The listing builds one solid part. Answer for the finished solid, in the listing's coordinates (mm). Face numbers are marked on the shaded views. A direction names the side the tool comes from. Give positions to 0.01 mm unless a question says otherwise; leave off trailing zeros. Loops run counter-clockwise (first coordinate to the right, second up) from the corner with the lowest first, then second, coordinate; pieces in that order, holes last. Notation, with made-up numbers: (58.5, 36.5) - (94.5, 36.5) arc R21 cw to (94.5, 75.5) - close; hole circle Ø8 at (62.25, -16.5). An arc over 180 degrees is marked (long way). Answer as CSV lines item,"result". Start each with the question number.
1) A cutting plane is placed at A-A (z = 13.5). Determine the outline of the cut face in (x, y).
2) Find the intervals of material crossed by line 1 along X through (y, z) = (-2, 17.5); line 2 along Z through (x, y) = (11, 22); line 3 along X through (y, z) = (-4, 10), in increasing order.
3) A cutting plane is placed at B-B (x = -12). Determine the outline of the cut face in (y, z), and give its area (3 significant figures).
4) For a pull along Y with two mould halves and no side action, classify the marked faces 1, 2 and 3 as pulls with the +Y half, pulls with the -Y half, needs draft (parallel to the pull), parting line crosses it, or undercut.
5) Flat-ended cylindrical pins translate along their axes: pin 1 (12.5 mm diameter, centred on x = 0, y = 0.19, fed in from +Z); pin 2 (1.5 mm diameter, centred on x = 12.5, y = -15, fed in from +Z); pin 3 (10 mm diameter, centred on y = -6, z = 6.5, fed in from -X); pin 4 (6 mm diameter, centred on x = 35, y = 0, fed in from +Z). Find the tip coordinate at first contact, or state that the pin passes through.
6) For the marked faces 4 and 5, determine the directions among +Z, -Z, +X, -X, +Y, -Y from which every point of the face is accessible in a straight line to the end or side of a thin tool.
7) A cutting plane is placed at D-D (x = -35). Determine the outline of the cut face in (y, z), and give its area (3 significant figures).
8) A cutting plane is placed at C-C (y = -11). Determine the outline of the cut face in (x, z), and give its area (3 significant figures).
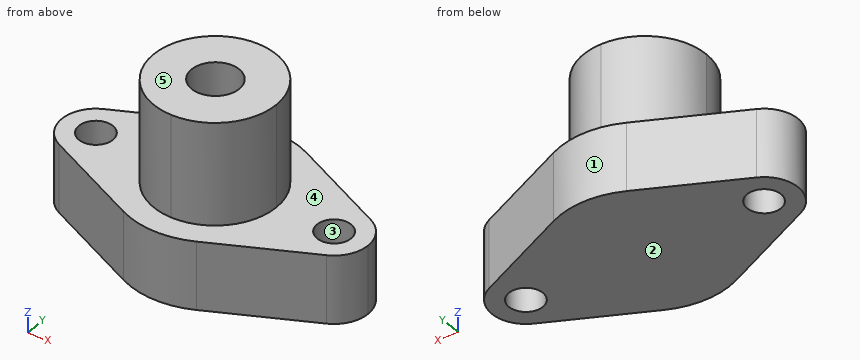
```python
from build123d import *

# Parameters (mm, degrees)
F1_DEPTH = 20
F3_D     = 10
F4_DEPTH = 30
F6_D     = 14
F6_DEPTH = 25
F6_TIP   = 4.2060243332


with BuildPart() as f1:
    # F0 (on Top) → F1 (new body)
    with BuildSketch(Plane.XY):
        with BuildLine():
            ThreePointArc((-25, 0), (-21.1288563682, 13.3630620956), (-10.7142857143, 22.5876975726))
            Line((-10.7142857143, 22.5876975726), (-39.2857142857, 9.0350790291))
            ThreePointArc((-39.2857142857, 9.0350790291), (-29.6547751618, 8.4515425473), (-25, 0))
        make_face()
        with BuildLine():
            Line((0, 0), (18, 0))
            ThreePointArc((18, 0), (0, 18), (-18, 0))
            Line((-18, 0), (0, 0))
        make_face()
        with BuildLine():
            Line((18, 0), (25, 0))
            ThreePointArc((25, 0), (21.1288563682, 13.3630620956), (10.7142857143, 22.5876975726))
            ThreePointArc((10.7142857143, 22.5876975726), (0, 25), (-10.7142857143, 22.5876975726))
            ThreePointArc((-10.7142857143, 22.5876975726), (-21.1288563682, 13.3630620956), (-25, 0))
            Line((-25, 0), (-18, 0))
            ThreePointArc((-18, 0), (0, 18), (18, 0))
        make_face()
        with BuildLine():
            ThreePointArc((-39.2857142857, -9.0350790291), (-29.6547751618, -8.4515425473), (-25, 0))
            ThreePointArc((-25, 0), (-29.6547751618, 8.4515425473), (-39.2857142857, 9.0350790291))
            ThreePointArc((-39.2857142857, 9.0350790291), (-45, 0), (-39.2857142857, -9.0350790291))
        make_face()
        with BuildLine():
            Line((-39.2857142857, -9.0350790291), (-10.7142857143, -22.5876975726))
            ThreePointArc((-10.7142857143, -22.5876975726), (-21.1288563682, -13.3630620956), (-25, 0))
            ThreePointArc((-25, 0), (-29.6547751618, -8.4515425473), (-39.2857142857, -9.0350790291))
        make_face()
        with BuildLine():
            ThreePointArc((39.2857142857, -9.0350790291), (29.6547751618, -8.4515425473), (25, 0))
            ThreePointArc((25, 0), (21.1288563682, -13.3630620956), (10.7142857143, -22.5876975726))
            Line((10.7142857143, -22.5876975726), (39.2857142857, -9.0350790291))
        make_face()
        with BuildLine():
            ThreePointArc((-18, 0), (0, -18), (18, 0))
            Line((18, 0), (0, 0))
            Line((0, 0), (-18, 0))
        make_face()
        with BuildLine():
            ThreePointArc((10.7142857143, -22.5876975726), (21.1288563682, -13.3630620956), (25, 0))
            Line((25, 0), (18, 0))
            ThreePointArc((18, 0), (0, -18), (-18, 0))
            Line((-18, 0), (-25, 0))
            ThreePointArc((-25, 0), (-21.1288563682, -13.3630620956), (-10.7142857143, -22.5876975726))
            ThreePointArc((-10.7142857143, -22.5876975726), (0, -25), (10.7142857143, -22.5876975726))
        make_face()
        with BuildLine():
            ThreePointArc((39.2857142857, 9.0350790291), (29.6547751618, 8.4515425473), (25, 0))
            ThreePointArc((25, 0), (29.6547751618, -8.4515425473), (39.2857142857, -9.0350790291))
            ThreePointArc((39.2857142857, -9.0350790291), (43.4515425473, -5.3452248382), (45, 0))
            ThreePointArc((45, 0), (43.4515425473, 5.3452248382), (39.2857142857, 9.0350790291))
        make_face()
        with BuildLine():
            ThreePointArc((10.7142857143, 22.5876975726), (21.1288563682, 13.3630620956), (25, 0))
            ThreePointArc((25, 0), (29.6547751618, 8.4515425473), (39.2857142857, 9.0350790291))
            Line((39.2857142857, 9.0350790291), (10.7142857143, 22.5876975726))
        make_face()
    extrude(amount=F1_DEPTH)

    # F3 (through all)
    with Locations(Plane(origin=(0, 0, 0), x_dir=(1, 0, 0), z_dir=(0, 0, -1))):
        with Locations((-35, 0), (35, 0)):
            Hole(F3_D / 2)

    # F2 (on face) → F4 (join)
    with BuildSketch(Plane.XY.offset(20)):
        with BuildLine():
            Line((0, -18), (0, 0))
            Line((0, 0), (-18, 0))
            ThreePointArc((-18, 0), (-12.7279220614, -12.7279220614), (0, -18))
        make_face()
        with BuildLine():
            Line((-18, 0), (0, 0))
            Line((0, 0), (0, 18))
            ThreePointArc((0, 18), (-12.7279220614, 12.7279220614), (-18, 0))
        make_face()
        with BuildLine():
            Line((0, 0), (18, 0))
            ThreePointArc((18, 0), (12.7279220614, 12.7279220614), (0, 18))
            Line((0, 18), (0, 0))
        make_face()
        with BuildLine():
            ThreePointArc((0, -18), (12.7279220614, -12.7279220614), (18, 0))
            Line((18, 0), (0, 0))
            Line((0, 0), (0, -18))
        make_face()
    extrude(amount=F4_DEPTH)

    # F6
    with Locations(Plane.XY.offset(50)):
        with Locations((0, 0.1870505988)):
            Hole(F6_D / 2, depth=F6_DEPTH)
            with Locations((0, 0, -(F6_DEPTH + F6_TIP / 2))):  # 118° drill point
                Cone(0, F6_D / 2, F6_TIP, mode=Mode.SUBTRACT)


solid = f1.part
```
Ans:
1,outline,"(-39.29, -9.04) - (-10.71, -22.59) arc R25 ccw to (10.71, -22.59) - (39.29, -9.04) arc R10 ccw to (39.29, 9.04) - (10.71, 22.59) arc R25 ccw to (-10.71, 22.59) - (-39.29, 9.04) arc R10 ccw to start; hole circle Ø10 at (-35, 0); hole circle Ø10 at (35, 0)"
2,line 1,"-44.8 to -39.58, -30.42 to 30.42, 39.58 to 44.8"
2,line 2,"0 to 20"
2,line 3,"-44.17 to -38, -32 to 32, 38 to 44.17"
3,outline,"(-21.98, 0) - (21.98, 0) - (21.98, 20) - (13.42, 20) - (13.42, 50) - (-13.42, 50) - (-13.42, 20) - (-21.98, 20) - close"
3,area,"1,680 mm2"
4,face 1,"pulls with the +Y half"
4,face 2,"needs draft"
4,face 3,"undercut"
5,pin 1,"z = 24.55"
5,pin 2,"z = 20"
5,pin 3,"x = -44.95"
5,pin 4,"through"
6,face 4,"+Z"
6,face 5,"+Z, +X, -X, +Y, -Y"
7,outline,"(-11.07, 0) - (-5, 0) - (-5, 20) - (-11.07, 20) - close; (5, 0) - (11.07, 0) - (11.07, 20) - (5, 20) - close"
7,area,"243 mm2"
8,outline,"(-35.14, 0) - (35.14, 0) - (35.14, 20) - (14.25, 20) - (14.25, 50) - (-14.25, 50) - (-14.25, 20) - (-35.14, 20) - close"
8,area,"2,260 mm2"
